Can you work these out from the model? Positions are in its coordinate system, mm. A direction names the side the tool comes from. Round coordinates to 2 decimals unless told otherwise and drop trailing zeros. Loops run counter-clockwise (first coordinate to the right, second up) from the corner with the lowest first, then second, coordinate; pieces in that order, holes last. Notation, with made-up numbers: (72, -5.5) -> (107, -5.5) arc R30 ccw to (107, 29.5) -> close; hole circle Ø9 at (17.5, 11). An arc over 180 degrees is marked (long way). Use a Markdown table: item, result.
from build123d import *

# Parameters (mm, degrees)
F0_W      = 90
F0_H      = 22
F1_DEPTH  = 10
F3_DEPTH  = 5
F4_R      = 2
F5_W      = 90
F5_H      = 22
F6_DEPTH  = 10
F8_DEPTH  = 10
F9_R      = 2
F11_DEPTH = 45
F13_DEPTH = 45
F14_R     = 2
F15_W     = 50
F15_H     = 22
F16_DEPTH = 10
F17_R     = 5
F18_DEPTH = 25
F18_TAPER = 3
F20_R     = 3
F21_DEPTH = 90
F22_R     = 2.5
F23_DEPTH = 3
F23_TAPER = 3
F24_R     = 2.5
F25_DEPTH = 3
F25_TAPER = 3


with BuildPart() as f1:
    # F0 (on Top) → F1 (new body)
    with BuildSketch(Plane.XY):
        with Locations((0, -55.5313304067)):
            Rectangle(F0_W, F0_H)
    extrude(amount=F1_DEPTH)

    # F2 (on face) → F3 (cut)
    with BuildSketch(Plane(origin=(0, 0, 0), x_dir=(1, 0, 0), z_dir=(0, 0, -1))):
        Polygon((-39.5, 44.5313304067), (0, 44.5313304067), (39.5, 44.5313304067), (39.19890013, 61.7813304067), (-39.19890013, 61.7813304067), align=None)
    extrude(amount=-F3_DEPTH, mode=Mode.SUBTRACT)

    # F4
    f4_edges = [f1.edges().sort_by_distance(p)[0] for p in [
        (-39.1989, -61.78133, 2.5),
        (39.1989, -61.78133, 2.5),
    ]]
    fillet(f4_edges, radius=F4_R)

    # F5 (on face) → F6 (join)
    with BuildSketch(Plane(origin=(0, 0, 0), x_dir=(1, 0, 0), z_dir=(0, 0, -1))):
        with Locations((0, 55.5313304067)):
            Rectangle(F5_W, F5_H)
    extrude(amount=F6_DEPTH)

    # F7 (on face) → F8 (cut)
    with BuildSketch(Plane(origin=(0, 0, -10), x_dir=(1, 0, 0), z_dir=(0, 0, -1))):
        Polygon((-20, 44.5313304067), (0, 44.5313304067), (20, 44.5313304067), (19.8167218183, 55.0313304067), (-19.8167218183, 55.0313304067), align=None)
        Polygon((19.8167218183, 55.0313304067), (20, 44.5313304067), (20, 55.0313304067), align=None)
        Polygon((-20, 55.0313304067), (-20, 44.5313304067), (-19.8167218183, 55.0313304067), align=None)
    extrude(amount=-F8_DEPTH, mode=Mode.SUBTRACT)

    # F9
    f9_edges = [f1.edges().sort_by_distance(p)[0] for p in [
        (-20, -55.03133, -5),
        (20, -55.03133, -5),
    ]]
    fillet(f9_edges, radius=F9_R)

    # F10 (on face) → F11 (join)
    with BuildSketch(Plane(origin=(0, 0, -10), x_dir=(1, 0, 0), z_dir=(0, 0, -1))):
        Polygon((-25, 44.5313304067), (0, 44.5313304067), (25, 44.5313304067), (25, 66.5313304067), (-25, 66.5313304067), align=None)
    extrude(amount=F11_DEPTH)

    # F12 (on face) → F13 (cut)
    with BuildSketch(Plane(origin=(0, 0, -55), x_dir=(1, 0, 0), z_dir=(0, 0, -1))):
        Polygon((-17.5, 44.5313304067), (0, 44.5313304067), (17.5, 44.5313304067), (17.3603594806, 52.5313304067), (-17.3603594806, 52.5313304067), align=None)
    extrude(amount=-F13_DEPTH, mode=Mode.SUBTRACT)

    # F14
    f14_edges = [f1.edges().sort_by_distance(p)[0] for p in [
        (-17.360359, -52.53133, -32.5),
        (17.360359, -52.53133, -32.5),
    ]]
    fillet(f14_edges, radius=F14_R)

    # F15 (on face) → F16 (join)
    with BuildSketch(Plane(origin=(0, 0, -55), x_dir=(1, 0, 0), z_dir=(0, 0, -1))):
        with Locations((0, 55.5313304067)):
            Rectangle(F15_W, F15_H)
    extrude(amount=F16_DEPTH)

    # F17 (on face) → F18 (cut)
    with BuildSketch(Plane(origin=(0, 0, -65), x_dir=(1, 0, 0), z_dir=(0, 0, -1))):
        with Locations((0, 44.5313304067)):
            Circle(F17_R)
    extrude(amount=-F18_DEPTH, taper=F18_TAPER, mode=Mode.SUBTRACT)

    # F20 (on face) → F21 (cut)
    with BuildSketch(Plane.XY.offset(10)):
        with Locations((22.7543748915, -44.5189550519)):
            Circle(F20_R)
        with Locations((-22.8854361922, -44.5189550519)):
            Circle(F20_R)
    extrude(amount=-F21_DEPTH, mode=Mode.SUBTRACT)

    # F22 (on face) → F23 (join)
    with BuildSketch(Plane(origin=(0, -44.5313304067, 0), x_dir=(-1, 0, 0), z_dir=(0, 1, 0))):
        with Locations((-15.0013593957, -60.537815094)):
            Circle(F22_R)
        with Locations((15.0013593957, -60.537815094)):
            Circle(F22_R)
    extrude(amount=F23_DEPTH, taper=F23_TAPER)

    # F24 (on face) → F25 (join)
    with BuildSketch(Plane(origin=(0, -44.5313304067, 0), x_dir=(-1, 0, 0), z_dir=(0, 1, 0))):
        with Locations((-42, 7.0607517846)):
            Circle(F24_R)
        with Locations((42, 7.0607517846)):
            Circle(F24_R)
    extrude(amount=F25_DEPTH, taper=F25_TAPER)


solid = f1.part
1. Which directions (+Z, -Z, +X, -X, +Y, -Y) give clear straight access to the entire face, cutting with the end or side of a thin tool? Please do faces 5 (the flat face through (-15, -41.531, -61)), 6 (the cylindrical face through (38.651, -61.193, 2.535)), 7 (the flat face through (35, -56, -10)), 8 (the flat face through (0, -44.531, 8)), 9 (the flat face through (-25, -56, -37)).
Answer sheet:
| item | result |
|---|---|
| face 5 | +Z, -Z, +X, -X, +Y |
| face 6 | +Y |
| face 7 | -Z, +X, +Y, -Y |
| face 8 | +Z, +Y |
| face 9 | -Z, -X, +Y, -Y |
2. I need wall thicknesses on line 1 (Z direction, x = 14, y = -47); line 2 (Z direction, x = -37, y = -52); line 3 (Z direction, x = 31.5, y = -64.75). Which ranges of each line are inside material? Lowest first, please.
Answer sheet:
| item | result |
|---|---|
| line 1 | z = -65 to -55, 5 to 10 |
| line 2 | z = -10 to 0, 5 to 10 |
| line 3 | z = -10 to 10 |
3. If we mould it in two halves opening along Z, with no side actions, what happens to faces 1 (the flat face through (15, -41.531, -61)), 2 (the conical face through (-44.309, -43.01, 7.788)), 3 (the flat face through (0, -56, -65)), 4 (the flat face through (-20, -49, -5))? For each: +Z half, -Z half, draft (parallel to the pull), parting line (faces both ways), or undercut.
Answer sheet:
| item | result |
|---|---|
| face 1 | draft |
| face 2 | parting line |
| face 3 | -Z half |
| face 4 | undercut |
4. I want a section at A-A (z = -6). Please give me the cut outline in (x, y), plus the area to 3 significant figures.
Answer sheet:
| item | result |
|---|---|
| outline | (-45, -66.53) -> (45, -66.53) -> (45, -44.53) -> (25.75, -44.53) arc R3 cw to (20, -45.71) -> (20, -53.03) arc R2 cw to (18, -55.03) -> (-18, -55.03) arc R2 cw to (-20, -53.03) -> (-20, -45.34) arc R3 cw to (-25.89, -44.53) -> (-45, -44.53) -> close |
| area | 1,530 mm² |
5. I want a section at B-B (x = 42). Please give me the cut outline in (y, z), plus the area to 3 significant figures.
Answer sheet:
| item | result |
|---|---|
| outline | (-66.53, -10) -> (-44.53, -10) -> (-44.53, 4.56) -> (-41.53, 4.72) -> (-41.53, 9.4) -> (-44.53, 9.56) -> (-44.53, 10) -> (-66.53, 10) -> close |
| area | 455 mm² |
6. Will these pins go through, and if not, where does the flat tip stop? pin 1 Ø7.5 at (x, z) = (-8.5, -42.5) entering from +Y; pin 2 Ø6 at (x, y) = (36, -59.5) entering from -Z; pin 3 Ø2 at (y, z) = (-56, -31.5) entering from +X.
Answer sheet:
| item | result |
|---|---|
| pin 1 | stops at y = -52.53 |
| pin 2 | stops at z = -10 |
| pin 3 | stops at x = 25 |
7. I want a section at D-D (z = -32.5). Please give me the cut outline in (x, y).
Answer sheet:
| item | result |
|---|---|
| outline | (-25, -66.53) -> (25, -66.53) -> (25, -46.51) arc R3 cw to (19.75, -44.53) -> (17.5, -44.53) -> (17.39, -50.57) arc R2 cw to (15.39, -52.53) -> (-15.39, -52.53) arc R2 cw to (-17.39, -50.57) -> (-17.5, -44.53) -> (-19.89, -44.53) arc R3 cw to (-25, -46.65) -> close |
8. I want a section at C-C (y = -63.75). Please give me the cut outline in (x, z).
Answer sheet:
| item | result |
|---|---|
| outline | (-45, -10) -> (-25, -10) -> (-25, -65) -> (25, -65) -> (25, -10) -> (45, -10) -> (45, 10) -> (-45, 10) -> close |
